Part model, mm, in its own coordinate system. A direction names the side the tool comes from. Round coordinates to 2 decimals unless told otherwise and drop trailing zeros. Loops run counter-clockwise (first coordinate to the right, second up) from the corner with the lowest first, then second, coordinate; pieces in that order, holes last. Notation, with made-up numbers: M 84.25,82 L 130.25,82 A19 ccw 130.25,118 Z; hole C 2.25,-9.5 d2. An arc over 180 degrees is marked long. Answer as CSV lines item,"result". Start each with the question number.
Item 1: Band-saw the part on A-A (z = -5.25). Give the cut face in (x, y).
Item 2: Which spindle directions (+Z, -Z, +X, -X, +Y, -Y) get a long thin tool onto all of the face, cutting with end or side? Do faces 5 (the flat face through (-61, 1, -2)), 6 (the flat face through (-151, -75, -1)). Say none if no direction does.
Item 3: Drop flat-ended pins along their axis: pin 1 Ø6 at (x, z) = (-14, -4) entering from -Y; pin 2 Ø2 at (x, z) = (39, -1) entering from -Y; pin 3 Ø1 at (x, y) = (-199.5, -16.5) entering from +Z. Give the stop position or say it passes through.
Item 4: Wall check: line 1 (Y direction, x = -153, z = -1.15); line 2 (X direction, y = -15, z = -1.5); line 3 (X direction, y = -44.5, z = -1.75). Give the ranges that are in metal, low to high.
Item 5: Band-saw the part on B-B (x = -64). Give the cut face in (y, z).
Item 6: Mould opens along Y. For faces 1 (the cylindrical face through (-199, -73, -19)), 2 (the cylindrical face through (-10, -35, -1)), 3 (the flat face through (-46.975, 65.367, -0.986)), 4 (the cylindrical face through (-10, 35, -1)) say: pulls with the +Y half, pulls with the -Y half, needs draft (parallel to the pull), parting line crosses it, or undercut.
Autodesk Inventor part; units mm, degrees
ref_plane "YZ Plane" through (0, 0, 0) normal (1, 0, 0) x (0, 1, 0)
ref_plane "XZ Plane" through (0, 0, 0) normal (0, 1, 0) x (-1, 0, 0)
ref_plane "XY Plane" through (0, 0, 0) normal (0, 0, 1) x (1, 0, 0)
ref_plane "Plano de trabajo1" through (0, 0, 0) normal (0, 0, 1) x (1, 0, 0)
sketch "Boceto1" plane through (0, 0, 0) normal (0, 0, 1) x (1, 0, 0)
  line L0 (75, -56) -> (80, -51)
  line L1 (80, -51) -> (80, 51)
  line L2 (80, 51) -> (75, 56)
  line L3 (75, 56) -> (-10, 56)
  line L4 (-10, 56) -> (-84.9998, 75)
  line L5 (-84.9998, 75) -> (-200, 75)
  line L6 (-200, 75) -> (-200, -75)
  line L7 (-200, -75) -> (-85, -75)
  line L8 (-85, -75) -> (-10.0003, -56)
  line L9 (-10.0003, -56) -> (75, -56)
  circle A0 centre (-184.9999, -70) radius 1.5
  circle A1 centre (25, -50) radius 1.5
  circle A2 centre (25, 50) radius 1.5
  line L10 (-91, 40) -> (-91, 59)
  arc A3 (-88, 62) -> (-91, 59) centre (-88, 59) ccw
  line L11 (-88, 62) -> (-74, 62)
  arc A4 (-71, 59) -> (-74, 62) centre (-74, 59) ccw
  line L12 (-71, 59) -> (-71, 40)
  arc A5 (-74, 37) -> (-71, 40) centre (-74, 40) ccw
  line L13 (-74, 37) -> (-88, 37)
  arc A6 (-91, 40) -> (-88, 37) centre (-88, 40) ccw
  line L14 (-91, -59) -> (-91, -40)
  arc A7 (-88, -37) -> (-91, -40) centre (-88, -40) ccw
  line L15 (-88, -37) -> (-74, -37)
  arc A8 (-71, -40) -> (-74, -37) centre (-74, -40) ccw
  line L16 (-71, -40) -> (-71, -59)
  arc A9 (-74, -62) -> (-71, -59) centre (-74, -59) ccw
  line L17 (-74, -62) -> (-88, -62)
  arc A10 (-91, -59) -> (-88, -62) centre (-88, -59) ccw
  line L18 (-20, -25) -> (-20, 25)
  line L19 (0, 25) -> (0, -25)
  circle A11 centre (-10, 25) radius 10
  circle A12 centre (-10, -25) radius 10
  circle A13 centre (-147.9, 65) radius 1.5
  circle A14 centre (-153, 39) radius 1.25
  circle A15 centre (-190, 15) radius 1.25
  circle A16 centre (-189.9, 0) radius 1.5
  circle A17 centre (-190, -43) radius 1.25
  circle A18 centre (-153, -19) radius 1.25
  circle A19 centre (-147.8999, -65) radius 1.5001
  circle A20 centre (-104, -43) radius 1.25
  circle A21 centre (-81.6553, -29) radius 1.25
  circle A22 centre (-104, -19) radius 1.25
  circle A23 centre (-32.6553, -29) radius 1.25
  circle A24 centre (-104, 15) radius 1.25
  circle A25 centre (-81.6553, 29) radius 1.25
  circle A26 centre (-104, 39) radius 1.25
  circle A27 centre (-32.6553, 29) radius 1.25
  circle A28 centre (4.1, -45) radius 1.5
  circle A29 centre (4, -20) radius 1.25
  circle A30 centre (12.6404, -20.8597) radius 1.5
  circle A31 centre (4, 20) radius 1.25
  circle A32 centre (12.6404, 20.8597) radius 1.5
  circle A33 centre (4.1, 45) radius 1.5
  circle A34 centre (54.6, -49.9999) radius 1.5001
  circle A35 centre (75, -50) radius 1.25
  circle A36 centre (75, -40) radius 1.25
  circle A37 centre (74, -28) radius 1.25
  circle A38 centre (54.3596, -20.8597) radius 1.5
  circle A39 centre (54.1, -9.25) radius 0.75
  circle A40 centre (40.1, -9.25) radius 0.75
  circle A41 centre (39.6, 50) radius 1.5
  circle A42 centre (54.6, 50) radius 1.5
  circle A43 centre (54.3597, 20.8596) radius 1.5
  circle A44 centre (54.1, 9.25) radius 0.75
  circle A45 centre (40.1, 9.25) radius 0.75
  circle A46 centre (74, 28) radius 1.25
  circle A47 centre (75, 50) radius 1.25
  circle A48 centre (75, 40) radius 1.25
  circle A49 centre (39.6, -50) radius 1.25
  circle A50 centre (25, -50) radius 1.5
  circle A51 centre (-95, -70) radius 1.5
  circle A52 centre (-185, -70) radius 1.5
  circle A53 centre (-185, 70) radius 1.5
  circle A54 centre (-95, 70) radius 1.5
  circle A55 centre (25, 50) radius 1.5
  point P0 (26.4595, -50.3464)
  point P1 (23.6185, -50.5842)
  point P2 (0, -24.9924)
  point P3 (-20, -24.9924)
extrude "Extrusión1" add sketch "Boceto1" against normal blind 2
ref_plane "Plano de trabajo2" through (-200, -75, -2.1) normal (-1, 0, 0) x (0, -1, 0)
sketch "Boceto2" plane through (-200, -75, -2.1) normal (-1, 0, 0) x (0, -1, 0)
  line L0 (-150, -12.9) -> (-150, 0.1)
  line L1 (-145, -17.9) -> (-5, -17.9)
  line L2 (-125, -8.4) -> (-25, -8.4)
  line L3 (-25, -15.4) -> (-125, -15.4)
  line L4 (-125, -15.4) -> (-125, -8.4)
  circle A0 centre (-130, -11.9) radius 1.5
  line L5 (-25, -8.4) -> (-25, -15.4)
  circle A1 centre (-20, -11.9) radius 1.5
  line L6 (0, -12.9) -> (0, 0.1)
  line L7 (0, 0.1) -> (-150, 0.1)
  arc A2 (-150, -12.9) -> (-145, -17.9) centre (-145, -12.9) ccw
  arc A3 (-5, -17.9) -> (0, -12.9) centre (-5, -12.9) ccw
  point P0 (-75, 2.1)
  dimension "d2" = 5
extrude "Extrusión2" add sketch "Boceto2" against normal blind 2
fillet "Empalme1" radius 2 1 edges at (-200, 0, 0)
properties part number "Base2"
Answer block:
1,outline,"M -200,-75 L -198,-75 L -198,75 L -200,75 Z"
2,face 5,"-Z, +X, +Y, -Y"
2,face 6,"+Z, -Z, +X, -X, -Y"
3,pin 1,"stops at y = -57.58"
3,pin 2,"stops at y = -56"
3,pin 3,"stops at z = -0.27"
4,line 1,"y = -75 to -20.25, -17.75 to 37.75, 40.25 to 75"
4,line 2,"x = -199.94 to -20, 0 to 80"
4,line 3,"x = -199.98 to -91, -71 to 2.69, 5.51 to 80"
5,outline,"M -69.68,-2 L 69.68,-2 L 69.68,0 L -69.68,0 Z"
6,face 1,"pulls with the -Y half"
6,face 2,"undercut"
6,face 3,"pulls with the +Y half"
6,face 4,"undercut"
